Autodesk Inventor part; units mm, degrees
ref_plane "YZ Plane" through (0, 0, 0) normal (1, 0, 0) x (0, 1, 0)
ref_plane "XZ Plane" through (0, 0, 0) normal (0, 1, 0) x (-1, 0, 0)
ref_plane "XY Plane" through (0, 0, 0) normal (0, 0, 1) x (1, 0, 0)
sketch "Sketch1" plane through (0, 0, 0) normal (0, 0, 1) x (1, 0, 0)
  arc A0 (33.1265, 11.2976) -> (-33.1265, 11.2976) centre (0, 0) ccw
  line L0 (-60, -67.5) -> (60, -67.5)
  line L1 (-60, -67.5) -> (-33.1265, 11.2976)
  line L2 (60, -67.5) -> (33.1265, 11.2976)
  point P0 (0, -67.5)
  dimension "d0" = 70
  dimension "d1" = 120
  dimension "d2" = 60
  dimension "d3" = 67.5
extrude "Extrusion1" add sketch "Sketch1" along normal blind 65
sketch "Sketch2" plane through (0, 0, 65) normal (0, 0, 1) x (1, 0, 0)
  circle A0 centre (0, 0) radius 35
  dimension "d6" = 70
extrude "Extrusion2" add sketch "Sketch2" along normal blind 25
sketch "Sketch3" plane through (0, 0, 90) normal (0, 0, 1) x (1, 0, 0)
  circle A0 centre (0, 0) radius 50
  dimension "d9" = 100
extrude "Extrusion3" add sketch "Sketch3" along normal blind 5
sketch "Sketch4" plane through (0, 0, 95) normal (0, 0, 1) x (1, 0, 0)
  circle A0 centre (0, -42.5) radius 3.75
  circle A1 centre (36.8061, 21.25) radius 3.75
  circle A2 centre (-36.8061, 21.25) radius 3.75
  point P0 (0, 0)
  dimension "d12" = 7.5
  dimension "d13" = 42.5
  dimension "d16" = 360
extrude "Extrusion4" cut sketch "Sketch4" against normal blind 5
sketch "Sketch5" plane through (0, 0, 90) normal (0, 0, -1) x (-1, 0, 0)
  line L0 (0, 60) -> (-30, 60)
  line L1 (-30, 60) -> (-30, 55.5)
  line L2 (-30, 55.5) -> (-25, 55.5)
  line L3 (-25, 55.5) -> (-25, 51)
  line L4 (-25, 51) -> (-30, 51)
  line L5 (-30, 51) -> (-30, 46.5)
  line L6 (-30, 46.5) -> (-25, 46.5)
  line L7 (-25, 46.5) -> (-25, 42)
  line L8 (-25, 42) -> (-30, 42)
  line L9 (-30, 42) -> (-30, 37.5)
  line L10 (-30, 37.5) -> (-25, 37.5)
  line L11 (-25, 37.5) -> (-25, 33)
  line L12 (-25, 33) -> (-30, 33)
  line L13 (-30, 33) -> (-30, 28.5)
  line L14 (-30, 28.5) -> (-25, 28.5)
  line L15 (-25, 28.5) -> (-25, 24)
  line L16 (-25, 24) -> (-30, 24)
  line L17 (-30, 24) -> (-30, 19.5)
  line L18 (-30, 19.5) -> (-25, 19.5)
  arc A0 (33.1265, 11.2976) -> (-33.1265, 11.2976) centre (0, 0) ccw
  line L19 (-25, 19.5) -> (0, 19.5)
  line L20 (0, 60) -> (30, 60)
  line L21 (30, 60) -> (30, 55.5)
  line L22 (30, 55.5) -> (25, 55.5)
  line L23 (25, 55.5) -> (25, 51)
  line L24 (25, 51) -> (30, 51)
  line L25 (30, 51) -> (30, 46.5)
  line L26 (30, 46.5) -> (25, 46.5)
  line L27 (25, 46.5) -> (25, 42)
  line L28 (25, 42) -> (30, 42)
  line L29 (30, 42) -> (30, 37.5)
  line L30 (30, 37.5) -> (25, 37.5)
  line L31 (25, 37.5) -> (25, 33)
  line L32 (25, 33) -> (30, 33)
  line L33 (30, 33) -> (30, 28.5)
  line L34 (30, 28.5) -> (25, 28.5)
  line L35 (25, 28.5) -> (25, 24)
  line L36 (25, 24) -> (30, 24)
  line L37 (30, 24) -> (30, 19.5)
  line L38 (30, 19.5) -> (25, 19.5)
  line L39 (25, 19.5) -> (0, 19.5)
  point P0 (0, 35)
  point P1 (-25, 24.4949)
  point P2 (25, 24.4949)
  dimension "d20" = 4.5
  dimension "d21" = 4.5
  dimension "d22" = 4.5
  dimension "d23" = 4.5
  dimension "d24" = 4.5
  dimension "d25" = 4.5
  dimension "d26" = 4.5
  dimension "d27" = 4.5
  dimension "d29" = 5
  dimension "d30" = 5
  dimension "d31" = 4.5
  dimension "d32" = 30
  dimension "d34" = 60
extrude "Extrusion5" add sketch "Sketch5" along normal blind 82.5 contours L20 L21 L22 L23 L24 L25 L26 L27 L28 L29 L30 L31 L32 L33 L34 L35 A0 L15 L14 L13 L12 L11 L10 L9 L8 L7 L6 L5 L4 L3 L2 L1 L0
sketch "Sketch6" plane through (0, 0, 95) normal (0, 0, 1) x (1, 0, 0)
  circle A0 centre (0, 0) radius 30
  dimension "d38" = 60
extrude "Extrusion6" cut sketch "Sketch6" against normal blind 90
sketch "Sketch7" plane through (0, 0, 5) normal (0, 0, 1) x (1, 0, 0)
  circle A0 centre (0, 0) radius 7.5
  dimension "d41" = 15
extrude "Extrusion7" cut sketch "Sketch7" against normal blind 90
properties part number "Base do Motor Industrial" material "Steel, Carbon"
Input: part model. Units: mm. Frame: model coordinates. A direction names the side the tool comes from. Coordinates: 2 decimals unless noted, no trailing zeros. Order: outer loops, then holes, each group sorted by start corner. A loop starts at its lowest first (then second) coordinate and runs counter-clockwise, first axis right, second up. Notation, with made-up numbers: M 49.25,24 L 75.25,24 A27 cw 75.25,56 Z; hole C 77.5,7.25 d7. An arc over 180 degrees is marked long. Write item = value, one per line. Start each with the question number.
(1) First-contact query: P1, Ø2, axis at y = 4.5, z = 22, coming from the -X side; P2, Ø1.3, axis at y = 45, z = 64.5, coming from the +X side; P3, Ø2, axis at y = 44.5, z = 51.5, coming from the -X side; P4, Ø13.5, axis at x = 0, y = 0, coming from the -Z side. Flat tips, straight axial feed; report the tip coordinate or a pass-through.
(2) Pull-direction query (Y, two-part tool) for faces 5 (the flat face through (-1, -67.5, 32)), 6 (the flat face through (28, 28.5, 49)), 7 (the flat face through (-30, 31, 49)); classes: released by +Y, released by -Y, zero draft, split by the parting line, or undercut.
(3) Section C-C on y = 0. Output: boundary loops of the cut face in (x, z), and give its area (3 significant figures).
(4) Reachability of faces 1 (the flat face through (27, 42, 49)), 2 (the flat face through (-25, 53, 49)), 3 (the flat face through (30, 58, 49)), 4 (the flat face through (-25, 44, 49)) from +Z, -Z, +X, -X, +Y, -Y: full face, straight path, thin tool, end or side. Return the list, or none.
(5) Section D-D on x = -45. Output: boundary loops of the cut face in (y, z).
(6) Section A-A on x = 0. Output: boundary loops of the cut face in (y, z).
(7) Line query: line 1 along Y through (x, z) = (0, 92.85); line 2 along Y through (x, z) = (0, 40.5); line 3 along Y through (x, z) = (0, 67.5). Output: solid intervals per line, ascending. Write a range as [from, to].
Result set:
q1.P1 = -35.79
q1.P2 = 25
q1.P3 = -25
q1.P4 = through
q2.face_5 = released by -Y
q2.face_6 = undercut
q2.face_7 = zero draft
q3.outline = M -50,90 L -35,90 L -35,65 L -36.98,65 L -36.98,0 L -7.5,0 L -7.5,5 L -30,5 L -30,95 L -50,95 Z; M 7.5,0 L 36.98,0 L 36.98,65 L 35,65 L 35,90 L 50,90 L 50,95 L 30,95 L 30,5 L 7.5,5 Z
q3.area = 1,580 mm²
q4.face_1 = -Z, +X
q4.face_2 = +Z, -Z, -X
q4.face_3 = +Z, -Z, +X, +Y
q4.face_4 = -Z, -X
q5.outline = M -67.5,0 L -23.52,0 L -23.52,65 L -67.5,65 Z; M -21.79,90 L 21.79,90 L 21.79,95 L -21.79,95 Z
q6.outline = M -67.5,0 L -7.5,0 L -7.5,5 L -30,5 L -30,95 L -38.75,95 L -38.75,90 L -35,90 L -35,65 L -67.5,65 Z; M -50,90 L -46.25,90 L -46.25,95 L -50,95 Z; M 7.5,0 L 35,0 L 35,7.5 L 60,7.5 L 60,90 L 50,90 L 50,95 L 30,95 L 30,5 L 7.5,5 Z
q7.line_1 = [-50, -46.25], [-38.75, -30], [30, 50]
q7.line_2 = [-67.5, -30], [30, 60]
q7.line_3 = [-35, -30], [30, 60]
